```python
from build123d import *

# Parameters (mm, degrees)
F1_DEPTH       = 304.8
F2_T1_DEPTH    = 33.0000735539
F4_D           = 3
F4_CBORE_D     = 10
F4_CBORE_DEPTH = 1
F5_R           = 6
F6_DEPTH       = 6


# Not quite as in the source:
# - a fillet or chamfer that OpenCascade refuses, or shapes differently, is made with other operations: its cross-section is extruded or revolved along the edge and cut away or added


with BuildPart() as f1:
    # F0 (on Top) → F1 (new body)
    with BuildSketch(Plane.XY):
        with BuildLine():
            ThreePointArc((-19.0469745753, -14.9999264461), (-33.9999816115, 0.0234873165), (-19, 15))
            Line((-19, 15), (0, 15))
            Line((0, 15), (19, 15))
            ThreePointArc((19, 15), (33.9999816115, 0.0234873165), (19.0469745753, -14.9999264461))
            ThreePointArc((19.0469745753, -14.9999264461), (19, -15), (18.9530254247, -14.9999264461))
            Line((18.9530254247, -14.9999264461), (15, -14.9999264461))
            Line((15, -14.9999264461), (15, -18))
            Line((15, -18), (19, -18))
            ThreePointArc((19, -18), (37, 0), (19, 18))
            Line((19, 18), (0, 18))
            Line((0, 18), (-19, 18))
            ThreePointArc((-19, 18), (-37, 0), (-19, -18))
            Line((-19, -18), (-15, -18))
            Line((-15, -18), (-15, -14.9999264461))
            Line((-15, -14.9999264461), (-18.9530254247, -14.9999264461))
            ThreePointArc((-18.9530254247, -14.9999264461), (-19, -15), (-19.0469745753, -14.9999264461))
        make_face()
    extrude(amount=F1_DEPTH)

    # F2: fillet of radius 15 on 2 edges, made by hand

    # F2_s2 → F2_t1 (cut)
    with BuildSketch(Plane.XZ.offset(-7.35539e-05)):
        with BuildLine():
            ThreePointArc((-30, 304.8), (-19.3933982822, 300.4066017178), (-15, 289.8))
            Line((-15, 289.8), (-14.7, 289.8))
            Line((-14.7, 289.8), (-14.7, 305.1))
            Line((-14.7, 305.1), (-30, 305.1))
            Line((-30, 305.1), (-30, 304.8))
        make_face()
        with BuildLine():
            ThreePointArc((30, 304.8), (19.3933982822, 300.4066017178), (15, 289.8))
            Line((15, 289.8), (14.7, 289.8))
            Line((14.7, 289.8), (14.7, 305.1))
            Line((14.7, 305.1), (30, 305.1))
            Line((30, 305.1), (30, 304.8))
        make_face()
    extrude(amount=F2_T1_DEPTH, mode=Mode.SUBTRACT)

    # F4 (through all)
    with Locations(Plane.XZ.offset(-15)):
        with Locations((0, 254.8), (0, 50)):
            CounterBoreHole(F4_D / 2, F4_CBORE_D / 2, F4_CBORE_DEPTH)

    # F5 (on face) → F6 (join)
    with BuildSketch(Plane(origin=(0, 0, 0), x_dir=(1, 0, 0), z_dir=(0, 0, -1))):
        with BuildLine():
            ThreePointArc((-19, 18), (-37, 0), (-19, -18))
            Line((-19, -18), (19, -18))
            ThreePointArc((19, -18), (37, 0), (19, 18))
            Line((19, 18), (-19, 18))
        make_face()
        with Locations((-19, 0)):
            Circle(F5_R, mode=Mode.SUBTRACT)
        with Locations((19, 0)):
            Circle(F5_R, mode=Mode.SUBTRACT)
    extrude(amount=F6_DEPTH)


solid = f1.part
```
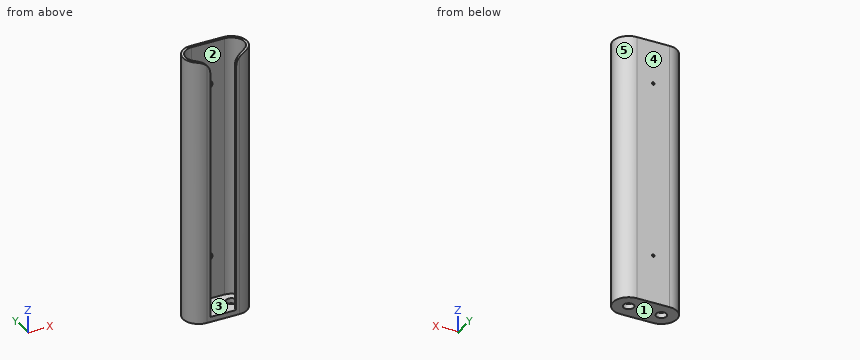
The listing builds one solid part. Answer for the finished solid, in the listing's coordinates (mm). Face numbers are marked on the shaded views. A direction names the side the tool comes from. Give positions to 0.01 mm unless a question says otherwise; leave off trailing zeros. Order: outer loops, then holes, each group sorted by start corner. A loop starts at its lowest first (then second) coordinate and runs counter-clockwise, first axis right, second up. Notation, with made-up numbers: (18.5, 13) -> (26.5, 13) arc R29 cw to (26.5, 38) -> close; hole circle Ø4 at (-22.75, -15). An arc over 180 degrees is marked (long way). One line per item, written item: value.
1) Find section A-A, the plane y = 0. Determine the outline of the cut face in (x, z), plus the area to 3 significant figures.
Reported:
outline: (-37, -6) -> (-25, -6) -> (-25, 0) -> (-34, 0) -> (-34, 304.8) -> (-37, 304.8) -> close; (-13, -6) -> (13, -6) -> (13, 0) -> (-13, 0) -> close; (25, -6) -> (37, -6) -> (37, 304.8) -> (34, 304.8) -> (34, 0) -> (25, 0) -> close
area: 2,130 mm^2
2) Determine the mould class of the marked faces 3, 4 and 5 for opening direction X: pulls with the +X half, pulls with the -X half, needs draft (parallel to the pull), parting line crosses it, or undercut.
Reported:
face 3: undercut
face 4: needs draft
face 5: pulls with the +X half
3) Find the intervals of material crossed by line 1 (Z direction, x = 0, y = 15.3); line 2 (Z direction, x = 0, y = 17.2); line 3 (X direction, y = 0, z = -1.35), in increasing order.
Reported:
line 1: z = -6 to 45, 55 to 249.8, 259.8 to 304.8
line 2: z = -6 to 48.5, 51.5 to 253.3, 256.3 to 304.8
line 3: x = -37 to -25, -13 to 13, 25 to 37
4) Find section C-C, the plane z = 126.5. Determine the outline of the cut face in (x, y), plus the area to 3 significant figures.
Reported:
outline: (-19.05, -15) arc R15 cw to (-19, 15) -> (19, 15) arc R15 cw to (19.05, -15) arc R15 cw to (18.95, -15) -> (15, -15) -> (15, -18) -> (19, -18) arc R18 ccw to (19, 18) -> (-19, 18) arc R18 ccw to (-19, -18) -> (-15, -18) -> (-15, -15) -> (-18.95, -15) arc R15 cw to start
area: 449 mm^2
5) Find section B-B, the plane x = -8. Determine the outline of the cut face in (y, z), plus the area to 3 significant figures.
Reported:
outline: (-18, -6) -> (18, -6) -> (18, 304.8) -> (15, 304.8) -> (15, 0) -> (-18, 0) -> close
area: 1,130 mm^2
6) Flat-ended cylindrical pins translate along their axes: P1, Ø1.5, axis at x = -5.5, y = 8.5, coming from the +Z side; P2, Ø3, axis at x = -1, z = 257, coming from the -Y side; P3, Ø2, axis at x = 6.5, z = 270.5, coming from the -Y side; P4, Ø10, axis at x = 20.5, z = 26.5, coming from the -Y side. Find the tip coordinate at first contact, or state that the pin passes through.
Reported:
P1: stops at z = 0
P2: stops at y = 16
P3: stops at y = 15
P4: stops at y = -18
7) A tool of negligible diameter and unlimited length cuts with its end or side. For the marked faces 1 and 2, from which of +Z, -Z, +X, -X, +Y, -Y can it reach the whole face along a straight path? Write none if from no direction.
Reported:
face 1: -Z, +X, -X, +Y, -Y
face 2: +Z
